```python
from build123d import *

# Parameters (mm, degrees)
CUT_EXTRUDE1_DEPTH      = 14.866731381
CUT_EXTRUDE1_DEPTH_BACK = 14.866731381
SKETCH2_R               = 1.5
SCALE1_SCALE            = 1.5


with BuildPart() as part:
    # Sketch1 → Revolve1 (revolve)
    with BuildSketch(Plane.XY, mode=Mode.PRIVATE) as revolve1_sk:
        with BuildLine():
            Line((-7, 8.712098042), (-7, 7.295703465))
            Line((-7, 7.295703465), (-7, 6.795703465))
            Line((-7, 6.795703465), (-7, 6.295703465))
            Line((-7, 6.295703465), (-7, 5.795703465))
            Line((-7, 5.795703465), (-7, -5.204296535))
            Line((-7, -5.204296535), (-6.25, -5.204296535))
            Line((-6.25, -5.204296535), (-5.050561785, -1.908867124))
            ThreePointArc((-5.050561785, -1.908867124), (-4.825715591, -1.069729704), (-4.75, -0.204296535))
            Line((-4.75, -0.204296535), (-4.75, 4.440083994))
            ThreePointArc((-4.75, 4.440083994), (-4.399873792, 5.550542455), (-3.476134386, 6.259352631))
            Line((-3.476134386, 6.259352631), (0, 7.524562078))
            Line((0, 7.524562078), (0, 8.566185983))
            Line((0, 8.566185983), (0, 9.69172121))
            add(Edge.make_bspline(
                [(-7, 8.712098042), (-6.915941705, 9.672888752), (-6.571850582, 9.786532429), (-6.017076444, 9.562037769), (-5.173496459, 8.320355176), (-3.929482137, 7.778040067), (-3.257853738, 7.770566701), (-1.62159895, 8.374478133), (-0.988089519, 9.078164836), (-0.514286955, 9.634062862), (-0.187546651, 9.695286605), (0, 9.69172121)],
                knots=[0, 0, 0, 0, 0.210746943, 0.254088111, 0.413486836, 0.459298403, 0.666392212, 0.714990212, 0.896680404, 0.92745251, 1, 1, 1, 1], degree=3))
        make_face()
    revolve(revolve1_sk.sketch.rotate(Axis((0, 2.420801252, 0), (0, 1, 0)), 270), axis=Axis((0, 2.420801252, 0), (0, 1, 0)))

    # Sketch2 → Cut-Extrude1 (cut, two sides: drawn at the far end of the back side and taken through both)
    with BuildSketch(Plane.XY.offset(-CUT_EXTRUDE1_DEPTH_BACK)):
        with Locations((0, 1.795703465)):
            Circle(SKETCH2_R)
    extrude(amount=CUT_EXTRUDE1_DEPTH + CUT_EXTRUDE1_DEPTH_BACK, mode=Mode.SUBTRACT)


with BuildPart() as part_1:
    # Scale1: scaled about (-7.054e-06, 3.062618866, 0.000522171)
    add(part.part.scale(SCALE1_SCALE).moved(Location((3.527e-06, -1.531309433, -0.000261085))))


solid = part_1.part
```
Here's how the part is built. I have some questions about the finished solid (model axes, mm). Coordinates: 2 decimals unless noted, no trailing zeros. Loops run counter-clockwise (first coordinate to the right, second up) from the corner with the lowest first, then second, coordinate; pieces in that order, holes last. Notation, with made-up numbers: (2, 25.5) - (23, 25.5) arc R23 cw to (23, 52.5) - close; hole circle Ø9 at (50.5, 35.5). An arc over 180 degrees is marked (long way). Return JSON: item names as keys, results as strings. Group by question number.
Item 1: I need wall thicknesses on line 1 (Z direction, x = -0.5, y = 10.75); line 2 (X direction, y = 11, z = 0.75); line 3 (Z direction, x = 4.25, y = -4). Which ranges of each line are inside material? Lowest first, please. Write a range as from..to.
Item 2: Will these pins go through, and if not, where does the flat tip stop? P1, Ø8.5, axis at x = 0, z = 0, coming from the +Y side; P2, Ø12, axis at x = -3.5, y = 9, coming from the +Z side; P3, Ø1.5, axis at y = -2, z = 7.5, coming from the -X side; P4, Ø2, axis at x = 7.5, y = 0, coming from the +Z side.
Item 3: If we section it at B-B on y = 9.25: Write out the boundary of the cut face in (x, z).
Item 4: If we section it at A-A on y = 4.5: Write out the boundary of the cut face in (x, z) (3 decimals), and give its area (3 significant figures).
Item 5: We'd pull the mould along Z, two halves only. Please class faces 1 (the face through (0.154, 9.663, 0.201)), 2 (the face through (-3.2, 1, -10)), 3 (the face through (2.73, 1.69, -6.58)), 4 (the face through (-9, -9.338, 4)): +Z half, -Z half, draft (parallel to the pull), parting line (faces both ways), or undercut.
Calculated:
{
 "1": {"line 1": "z = -10.49..-7.19, -3.21..3.21, 7.19..10.49", "line 2": "x = -10.47..-7.49, -2.68..2.68, 7.49..10.47", "line 3": "z = -9.6..-6.11, 6.11..9.6"},
 "2": {"P1": "stops at y = 13.01", "P2": "stops at z = 10.5", "P3": "stops at x = -8.04", "P4": "stops at z = 8.25"},
 "3": {"outline": "circle Ø21 at (0, 0); hole circle Ø2.78 at (0, 0)"},
 "4": {"outline": "circle Ø21 at (0, 0); hole circle Ø14.25 at (0, 0)", "area": "187 mm^2"},
 "5": {"face 1": "undercut", "face 2": "parting line", "face 3": "undercut", "face 4": "draft"}
}
